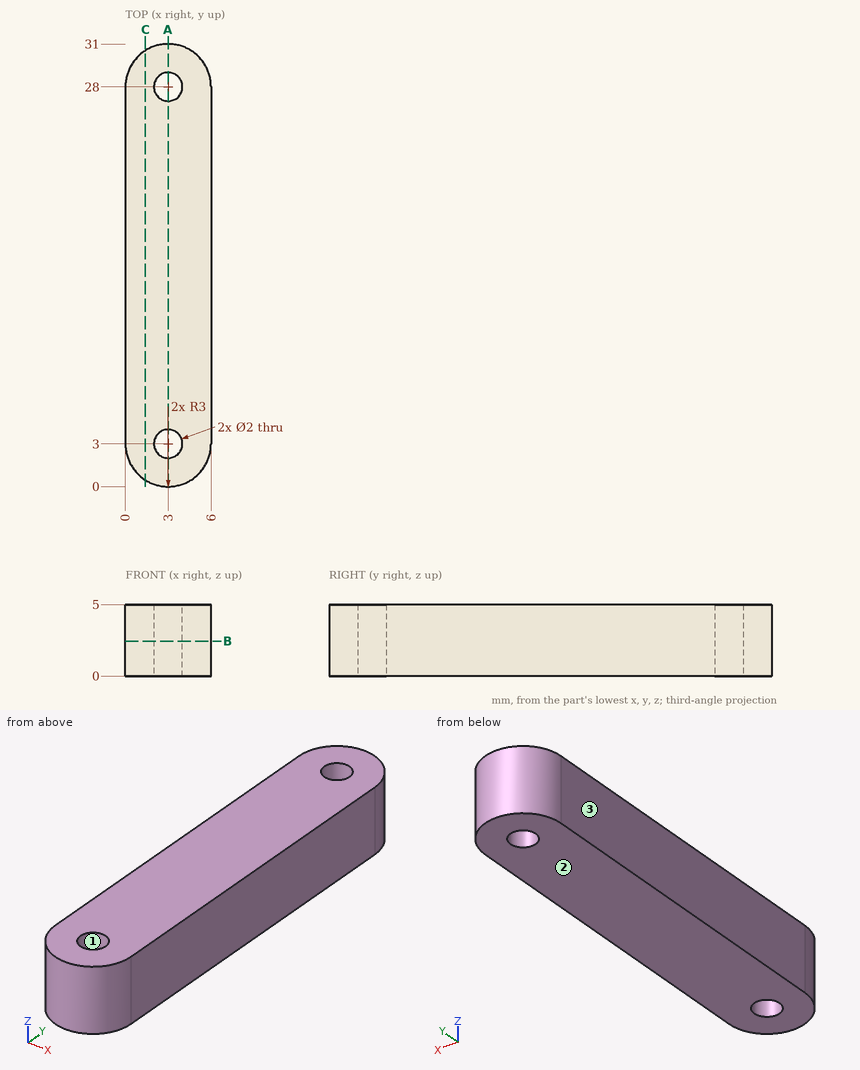
Job drawing, mm, ordinate dimensions from the low corner. One solid piece. Coordinates: 2 decimals unless noted, no trailing zeros. Order: outer loops, then holes, each group sorted by start corner. A loop starts at its lowest first (then second) coordinate and runs counter-clockwise, first axis right, second up. Notation, with made-up numbers: (71.5, 23) -> (93.5, 23) arc R23 cw to (93.5, 51) -> close; hole circle Ø6 at (-20.5, 43). An arc over 180 degrees is marked (long way). Put each result on its own line as item: value. Start each with the question number.
(1) Band-saw the part on C-C (x = 1.4). Give the cut face in (y, z), then the cut area to 3 significant figures.
(2) Probe line 1 along Y through (x, z) = (3, 2.7); line 2 along Y through (x, z) = (2.3, 0.8); line 3 along Y through (x, z) = (0.45, 0.9). List the from-to ranges inside material, lowest first. Write a range as [from, to].
(3) Band-saw the part on A-A (x = 3). Give the cut face in (y, z).
(4) Mould opens along X. For the marked faces 1, 2 and 3 say: pulls with the +X half, pulls with the -X half, needs draft (parallel to the pull), parting line crosses it, or undercut.
(5) Band-saw the part on B-B (z = 2.45). Give the cut face in (x, y).
Determined:
1. outline: (0.46, 0) -> (30.54, 0) -> (30.54, 5) -> (0.46, 5) -> close
1. area: 150 mm²
2. line 1: y = [0, 2], [4, 27], [29, 31]
2. line 2: y = [0.08, 2.29], [3.71, 27.29], [28.71, 30.92]
2. line 3: y = [1.42, 29.58]
3. outline: (0, 0) -> (2, 0) -> (2, 5) -> (0, 5) -> close; (4, 0) -> (27, 0) -> (27, 5) -> (4, 5) -> close; (29, 0) -> (31, 0) -> (31, 5) -> (29, 5) -> close
4. face 1: undercut
4. face 2: needs draft
4. face 3: pulls with the -X half
5. outline: (0, 3) arc R3 ccw to (6, 3) -> (6, 28) arc R3 ccw to (0, 28) -> close; hole circle Ø2 at (3, 3); hole circle Ø2 at (3, 28)
